Build history of the part. All positions in model axes, mm. A direction names the side the tool comes from. Round coordinates to 2 decimals unless told otherwise and drop trailing zeros. Loops run counter-clockwise (first coordinate to the right, second up) from the corner with the lowest first, then second, coordinate; pieces in that order, holes last. Notation, with made-up numbers: (-7.75, -2.5) - (11.25, -2.5) arc R22 cw to (11.25, 16.5) - close; hole circle Ø5 at (5, 11.5). An arc over 180 degrees is marked (long way). Put each result on its own line as item: value. Start each with the question number.
from build123d import *

# Parameters (mm, degrees)
F0_R     = 4.25
F1_DEPTH = 17
F2_DEPTH = 5
F4_DEPTH = 12
F5_W     = 4.6458135775
F5_H     = 1.5
F5_W_2   = 3.3541864225
F5_W_3   = 8
F6_DEPTH = 40
F7_R     = 12.5
F7_R_2   = 4.25
F8_DEPTH = 6


# Not quite as in the source:
# - a feature names something its author has since deleted; it is built from what else it names


with BuildPart() as f1:
    # F0 (on Front) → F1 (new body)
    with BuildSketch(Plane.XZ):
        with BuildLine():
            ThreePointArc((-8.5, -5.4772255751), (-8.5266357667, -5.2791241211), (-8.6046511628, -5.0950935582))
            ThreePointArc((-8.6046511628, -5.0950935582), (-9.9967746616, -5.5467065419), (-8.5452305344, -5.7337406825))
            ThreePointArc((-8.5452305344, -5.7337406825), (-8.5113941852, -5.6074617083), (-8.5, -5.4772255751))
        make_face()
        with BuildLine():
            ThreePointArc((-8.6046511628, -5.0950935582), (0, 10), (8.6046511628, -5.0950935582))
            ThreePointArc((8.6046511628, -5.0950935582), (9.4481014539, -4.7538613418), (10, -5.4772255751))
            ThreePointArc((10, -5.4772255751), (9.3802361333, -6.2158313898), (8.5452305344, -5.7337406825))
            Line((8.5452305344, -5.7337406825), (12.6458135775, -17))
            Line((12.6458135775, -17), (16, -17))
            Line((16, -17), (16, 65))
            Line((16, 65), (-16, 65))
            Line((-16, 65), (-16, -17))
            Line((-16, -17), (-12.6458135775, -17))
            Line((-12.6458135775, -17), (-8.5452305344, -5.7337406825))
            ThreePointArc((-8.5452305344, -5.7337406825), (-9.9967746616, -5.5467065419), (-8.6046511628, -5.0950935582))
        make_face()
        with Locations((0, 42.5)):
            Circle(F0_R, mode=Mode.SUBTRACT)
        with BuildLine():
            ThreePointArc((10, -5.4772255751), (9.4481014539, -4.7538613418), (8.6046511628, -5.0950935582))
            ThreePointArc((8.6046511628, -5.0950935582), (8.5032253384, -5.4077446082), (8.5452305344, -5.7337406825))
            ThreePointArc((8.5452305344, -5.7337406825), (9.3802361333, -6.2158313898), (10, -5.4772255751))
        make_face()
    extrude(amount=F1_DEPTH)

    # F0 (on Front) → F2 (join)
    with BuildSketch(Plane.XZ):
        with BuildLine():
            ThreePointArc((8.5452305344, -5.7337406825), (8.5032253384, -5.4077446082), (8.6046511628, -5.0950935582))
            ThreePointArc((8.6046511628, -5.0950935582), (0, 10), (-8.6046511628, -5.0950935582))
            ThreePointArc((-8.6046511628, -5.0950935582), (-8.5266357667, -5.2791241211), (-8.5, -5.4772255751))
            ThreePointArc((-8.5, -5.4772255751), (-8.5113941852, -5.6074617083), (-8.5452305344, -5.7337406825))
            Line((-8.5452305344, -5.7337406825), (-12.6458135775, -17))
            Line((-12.6458135775, -17), (-4.5, -17))
            Line((-4.5, -17), (-4.5, 0))
            ThreePointArc((-4.5, 0), (0, 4.5), (4.5, 0))
            Line((4.5, 0), (4.5, -17))
            Line((4.5, -17), (12.6458135775, -17))
            Line((12.6458135775, -17), (8.5452305344, -5.7337406825))
        make_face()
    extrude(amount=F2_DEPTH)

    # F3 (on face) → F4 (cut)
    with BuildSketch(Plane.XZ.offset(17)):
        with BuildLine():
            Line((-8.6046511628, 23), (-8.6046511628, 5.0950935582))
            ThreePointArc((-8.6046511628, 5.0950935582), (-8.0458244358, 5.938409648), (-7.4046511628, 6.7209479359))
            Line((-7.4046511628, 6.7209479359), (-7.4046511628, 23))
            Line((-7.4046511628, 23), (-8.6046511628, 23))
        make_face()
        with BuildLine():
            Line((7.4046511628, 23), (7.4046511628, 6.7209479359))
            ThreePointArc((7.4046511628, 6.7209479359), (8.0458244358, 5.938409648), (8.6046511628, 5.0950935582))
            Line((8.6046511628, 5.0950935582), (8.6046511628, 23))
            Line((8.6046511628, 23), (7.4046511628, 23))
        make_face()
    extrude(amount=-F4_DEPTH, mode=Mode.SUBTRACT)

    # F5 (on face) → F6 (cut)
    with BuildSketch(Plane(origin=(0, 0, -17), x_dir=(1, 0, 0), z_dir=(0, 0, -1))):
        with Locations((-10.3229067887, 5.75)):
            Rectangle(F5_W, F5_H)
        with Locations((-14.3229067887, 5.75)):
            Rectangle(F5_W_2, F5_H)
        with Locations((12, 5.75)):
            Rectangle(F5_W_3, F5_H)
    extrude(amount=-F6_DEPTH, mode=Mode.SUBTRACT)

    # F7 (on face) → F8 (cut)
    with BuildSketch(Plane.XZ.offset(17)):
        with Locations((0, 42.5)):
            Circle(F7_R)
        with Locations((0, 42.5)):
            Circle(F7_R_2, mode=Mode.SUBTRACT)
    extrude(amount=-F8_DEPTH, mode=Mode.SUBTRACT)


solid = f1.part
Item 1: Slice it at B-B (z = 42.5). Give the cut face in (x, y).
Item 2: Drop flat-ended pins along their axis: pin 1 Ø12 at (x, z) = (-8, 12) entering from +Y; pin 2 Ø9.5 at (x, z) = (-4.5, -2) entering from -Y; pin 3 Ø7.5 at (x, z) = (1, 43) entering from -Y. Give the stop position or say it passes through.
Item 3: Two-plate mould, pull along X, no slides. Class faces 6 (the flat face through (-16, -8, 25)), 7 (the flat face through (0, -8, 65)), 8 (the flat face through (-4.5, -2, -9)): pulls with the +X half, pulls with the -X half, needs draft (parallel to the pull), parting line crosses it, or undercut.
Item 4: Slice it at D-D (z = 6). Give the cut face in (x, y), plus the area to 3 significant figures.
Item 5: Slice it at C-C (y = -8.25). Give the cut face in (x, z), plus the area to 3 significant figures.
Item 6: Slice it at A-A (x = 0). Give the cut face in (y, z), plus the area to 3 significant figures.
Item 7: Drill centre lines: probe 1 along X at (y, z) = (-9, 17); probe 2 along Z at (x, y) = (0, -13.8); probe 3 along Y at (x, z) = (10, 10.5). Where is each one in solid material? Low to high. Write a range as [from, to].
Item 8: Which spindle directions (+Z, -Z, +X, -X, +Y, -Y) get a long thin tool onto all of the face, cutting with end or side? Do faces 1 (the flat face through (7.405, -11, 15)), 2 (the flat face through (0, -11, 37)), 3 (the flat face through (4.5, -2, -8)), 4 (the flat face through (12, -6.5, 3)), 5 (the flat face through (-14, -12, -17)). Say none if no direction does.
Computed values:
1. outline: (-16, -17) - (-12.5, -17) - (-12.5, -11) - (-4.25, -11) - (-4.25, 0) - (-16, 0) - close; (4.25, -11) - (12.5, -11) - (12.5, -17) - (16, -17) - (16, 0) - (4.25, 0) - close
2. pin 1: stops at y = 0
2. pin 2: stops at y = -5
2. pin 3: stops at y = -11
3. face 6: pulls with the -X half
3. face 7: needs draft
3. face 8: undercut
4. outline: (-16, -17) - (-8.6, -17) - (-8.6, -6.5) - (-16, -6.5) - close; (-16, -5) - (16, -5) - (16, 0) - (-16, 0) - close; (8.6, -17) - (16, -17) - (16, -6.5) - (8.6, -6.5) - close
4. area: 315 mm^2
5. outline: (-16, -17) - (-12.65, -17) - (-8.55, -5.73) arc R0.75 ccw to (-8.6, -5.1) arc R10 cw to (-8.6, 5.1) - (-8.6, 23) - (-7.4, 23) - (-7.4, 6.72) arc R10 cw to (7.4, 6.72) - (7.4, 23) - (8.6, 23) - (8.6, 5.1) arc R10 cw to (8.6, -5.1) arc R0.75 ccw to (8.55, -5.73) - (12.65, -17) - (16, -17) - (16, 65) - (-16, 65) - close; hole circle Ø8.5 at (0, 42.5)
5. area: 2,020 mm^2
6. outline: (-17, 10) - (-5, 10) - (-5, 4.5) - (0, 4.5) - (0, 38.25) - (-11, 38.25) - (-11, 30) - (-17, 30) - close; (-17, 55) - (-11, 55) - (-11, 46.75) - (0, 46.75) - (0, 65) - (-17, 65) - close
6. area: 719 mm^2
7. probe 1: x = [-16, -8.6], [-7.4, 7.4], [8.6, 16]
7. probe 2: z = [10, 30], [55, 65]
7. probe 3: y = [-17, -6.5], [-5, 0]
8. face 1: -Z, -Y
8. face 2: -Y
8. face 3: -Z, +Y, -Y
8. face 4: -Z, +X
8. face 5: -Z, +X, -X, +Y, -Y
